Design review of the part built by this model. Coordinates are the model's own, in mm. A direction names the side the tool comes from. Coordinates: 2 decimals unless noted, no trailing zeros. Write each loop counter-clockwise with the first axis right and the second up, starting at its lowest first coordinate (ties: lowest second). Pieces come first, ordered by that corner, then holes.
Q1. The part is to be moulded in two halves that separate along Y. For faces 1 (the flat face through (396, 318, 495)), 2 (the flat face through (800, 433, 449)), 3 (the flat face through (82.906, 25.358, 448.534)), say which applies: released by +Y, released by -Y, zero draft, split by the parting line, or undercut.
Q2. For pin 1 Ø19.5 at (x, y) = (297.5, 26) entering from -Z; pin 2 Ø4 at (x, z) = (513.5, 87) entering from +Y, all flat-tipped, find the tip position at first contact; note any pin that passes through.
Q3. Take a section at D-D, the plane y = 261. Write out the cut boundary in (x, z), plus the area to 3 significant figures.
Q4. For faces 4 (the flat face through (405, 20, 370)), 5 (the flat face through (715.987, 277.074, 270.495)), 6 (the flat face through (406, 600, 370)), list the 3-axis set-ups (+Z, -Z, +X, -X, +Y, -Y) from which the entire face can be reached by the end or side of a thin tool; tool diameter is ignored.
Q5. Take a section at C-C, the plane z = 55. Write out the cut boundary in (x, y).
Q6. For L1, parallel to Z at x = 618.5, y = 311; L2, parallel to Z at x = 344.5, y = 165; L3, parallel to X at y = 283.5, z = 459, list the stretches that pass through material, from the lowest coordinate up.
Q7. Take a section at A-A, the plane x = 345.5. Write out the cut boundary in (y, z), plus the area to 3 significant figures.
Q8. Take a section at B-B, the plane y = 457. Write out the cut boundary in (x, z).
Autodesk Inventor part; units mm, degrees
ref_plane "YZ Plane" through (0, 0, 0) normal (1, 0, 0) x (0, 1, 0)
ref_plane "XZ Plane" through (0, 0, 0) normal (0, 1, 0) x (-1, 0, 0)
ref_plane "XY Plane" through (0, 0, 0) normal (0, 0, 1) x (1, 0, 0)
sketch "Sketch1" plane through (0, 0, 0) normal (0, 0, 1) x (1, 0, 0)
  line L0 (130, 0) -> (670, 0)
  line L1 (800, 70) -> (800, 620)
  line L2 (800, 620) -> (0, 620)
  line L3 (0, 620) -> (0, 70)
  line L4 (0, 70) -> (130, 0)
  line L5 (670, 0) -> (800, 70)
  line L6 (400, 620) -> (400, 0) construction
  point P0 (0, 0)
  dimension "d0" = 800
  dimension "d1" = 620
  dimension "d2" = 550
  dimension "d3" = 550
  dimension "d4" = 270
  dimension "d5" = 270
  dimension "d6" = 70
  dimension "d7" = 70
  dimension "d8" = 130
  dimension "d9" = 130
extrude "Extrusion1" add sketch "Sketch1" along normal blind 500
sketch "Sketch2" plane through (800, 70, 0) normal (1, 0, 0) x (0, 0, -1)
  line L0 (-370, -31) -> (0, 80)
  line L1 (0, 80) -> (0, -70)
  line L2 (0, -70) -> (-370, -70)
  line L3 (0, 550) -> (-500, 550)
  line L4 (-370, 511) -> (0, 400)
  line L5 (0, 400) -> (0, 550)
  line L6 (0, 550) -> (-370, 550)
  line L7 (-370, -31) -> (-370, -70)
  line L8 (0, -70) -> (-500, -70)
  line L9 (-370, 511) -> (-370, 550)
  line L10 (-500, -70) -> (-500, 0)
  line L11 (-500, 0) -> (-500, 550)
  dimension "d12" = 320
  dimension "d15" = 150
  dimension "d16" = 150
  dimension "d17" = 130
  dimension "d18" = 130
extrude "Extrusion2" cut sketch "Sketch2" against normal through all
sketch "Sketch3" plane through (0, 0, 500) normal (0, 0, 1) x (1, 0, 0)
  line L0 (125, 520) -> (675, 520)
  line L1 (675, 520) -> (675, 110)
  line L2 (675, 110) -> (125, 110)
  line L3 (125, 110) -> (125, 520)
  line L4 (800, 620) -> (0, 620)
  line L5 (0, 150) -> (0, 470)
  line L6 (800, 70) -> (800, 620)
  point P0 (0, 0)
  dimension "d21" = 100
  dimension "d22" = 125
  dimension "d23" = 125
  dimension "d24" = 40
  dimension "d33" = 550
  dimension "d34" = 410
extrude "Extrusion3" cut sketch "Sketch3" against normal blind 5
sketch "Sketch4" plane through (0, 581, 370) normal (0, 0.9578, -0.2873) x (1, 0, 0)
  line L0 (800, 0) -> (0, 0)
  line L1 (800, 0) -> (580, 478.2427)
  line L2 (800, 478.2427) -> (0, 478.2427)
  line L3 (0, 0) -> (220, 478.2427)
  line L4 (220, 478.2427) -> (0, 478.2427)
  line L5 (800, -11.2066) -> (0, -11.2066)
  line L6 (0, 0) -> (0, 386.2913)
  line L7 (0, 478.2427) -> (0, 0)
  line L8 (800, 0) -> (800, 478.2427)
  line L9 (800, 245.8102) -> (800, 22.3174)
  line L10 (800, 478.2427) -> (580, 478.2427)
  point P0 (0, 521.3448)
  dimension "d27" = 360
  dimension "d28" = 220
  dimension "d30" = 220
extrude "Extrusion4" cut sketch "Sketch4" against normal through all contours L1 L2 L8 | L6 L7 L2 L3
properties part number "TV" material "ABS Plastic"
Responses:
1. face 1: undercut
1. face 2: zero draft
1. face 3: released by -Y
2. pin 1: stops at z = 370
2. pin 2: stops at y = 496.7
3. outline: (0, 465.99) - (205.32, 0) - (594.68, 0) - (800, 465.99) - (800, 500) - (675, 500) - (675, 495) - (125, 495) - (125, 500) - (0, 500) - close
3. area: 302,000 mm2
4. face 4: -Z, +X, -X, -Y
4. face 5: -Z, +X, -Y
4. face 6: -Z, +X, -X, +Y
5. outline: (151.29, 486.5) - (197.94, 133.5) - (602.06, 133.5) - (648.71, 486.5) - close
6. L1: z = 39.07 to 495
6. L2: z = 0 to 495
6. L3: x = 0.1 to 799.9
7. outline: (0, 370) - (39, 370) - (150, 0) - (470, 0) - (581, 370) - (620, 370) - (620, 500) - (520, 500) - (520, 495) - (110, 495) - (110, 500) - (0, 500) - close
7. area: 238,000 mm2
8. outline: (0, 407.19) - (179.42, 0) - (620.58, 0) - (800, 407.19) - (800, 500) - (675, 500) - (675, 495) - (125, 495) - (125, 500) - (0, 500) - close
